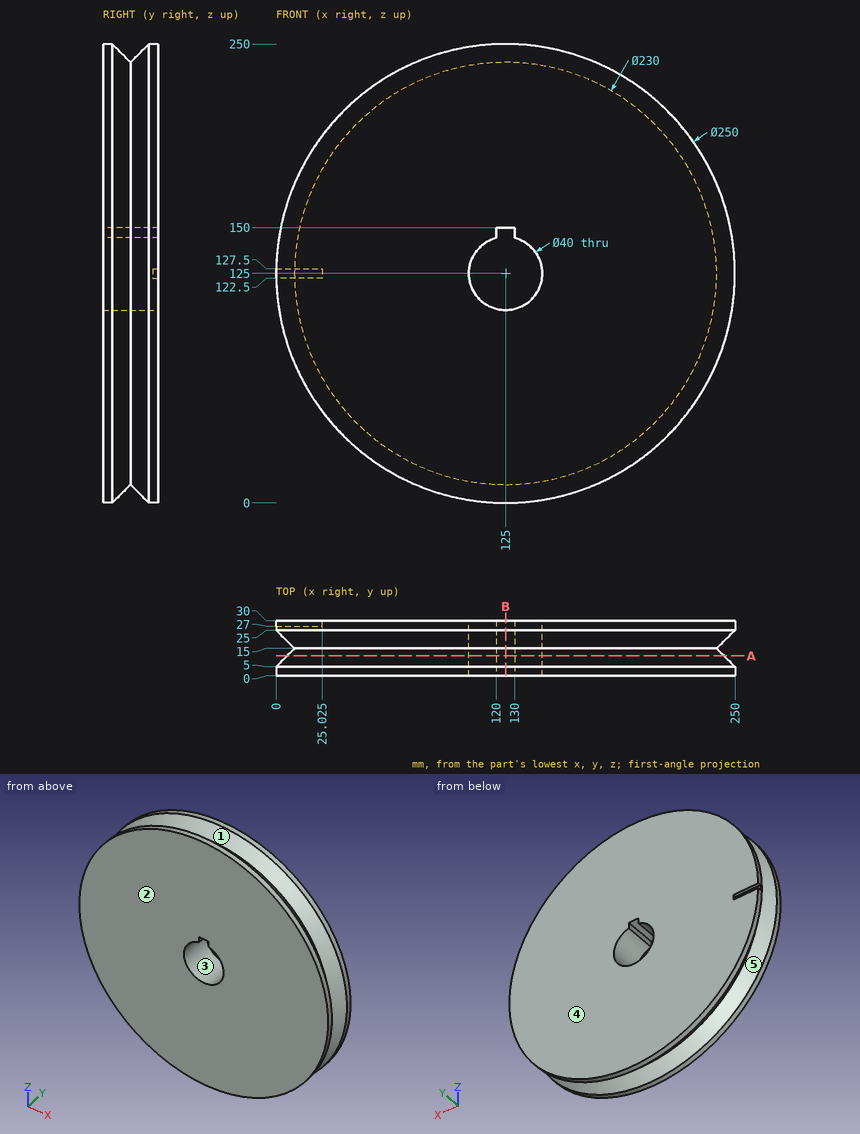
Geometry: see drawing. Coordinates: mm, zero at the bounding-box minimum. A direction names the side the tool comes from. Give positions to 0.01 mm unless a question says otherwise; leave off trailing zeros. Order: outer loops, then holes, each group sorted by start corner. A loop starts at its lowest first (then second) coordinate and runs counter-clockwise, first axis right, second up. Notation, with made-up numbers: M -23,79 L 6,79 A10 cw 6,91 Z; hole C 13.25,45.5 d6. An arc over 180 degrees is marked long. Answer as a JSON object with one key per item and string values.
1. First-contact query: P1, Ø4, axis at x = 200.5, y = 9, coming from the -Z side; P2, Ø1, axis at x = 72.5, y = 23, coming from the +Z side; P3, Ø0.9, axis at x = 12, y = 28, coming from the +Z side. Flat tips, straight axial feed; report the tip coordinate or a pass-through.
Result sheet:
{"P1": "z = 27.47", "P2": "z = 236.83", "P3": "z = 179.38"}
2. Ray query, line 1 (Z direction, x = 125, y = 17.5); line 2 (Z direction, x = 125, y = 11.25); line 3 (X direction, y = 11.75, z = 146). Return the intervals inside material, ascending. Write a range as [from, to].
Result sheet:
{"line 1": "[7.5, 105], [150, 242.5]", "line 2": "[6.25, 105], [150, 243.75]", "line 3": "[8.63, 120], [130, 241.37]"}
3. Pull-direction query (X, two-part tool) for the marked faces 3, 4 and 5; classes: +X half, -X half, draft (parallel to the pull), parting line (faces both ways), or undercut.
Result sheet:
{"face 3": "undercut", "face 4": "draft", "face 5": "parting line"}
4. Cut plane B-B, the plane x = 125. Output: boundary loops of the cut face in (y, z), and give its area (3 significant figures).
Result sheet:
{"outline": "M 0,0 L 5,0 L 15,10 L 25,0 L 30,0 L 30,105 L 0,105 Z; M 0,150 L 30,150 L 30,250 L 25,250 L 15,240 L 5,250 L 0,250 Z", "area": "5,950 mm²"}
5. Reachability of the marked faces 1 and 2 from +Z, -Z, +X, -X, +Y, -Y: full face, straight path, thin tool, end or side. Return the list, or none.
Result sheet:
{"face 1": "none", "face 2": "+Z, -Z, +X, -X, -Y"}
6. Cut plane A-A, the plane y = 11. Output: boundary loops of the cut face in (x, z), and give its area (3 significant figures).
Result sheet:
{"outline": "C 125,125 d238; hole M 120,144.36 A20 ccw long 130,144.36 L 130,150 L 120,150 Z", "area": "43,200 mm²"}
